Could you check a few things on this model? Use its own coordinates, in mm. Face numbers are marked on the shaded views. A direction names the side the tool comes from. Coordinates: 2 decimals unless noted, no trailing zeros. Loops run counter-clockwise (first coordinate to the right, second up) from the corner with the lowest first, then second, coordinate; pieces in that order, holes last. Notation, with made-up numbers: (-8, 87.5) - (36, 87.5) arc R9 ccw to (36, 95.5) - close; hole circle Ø9 at (29, -38.75). An arc over 180 degrees is marked (long way). Put each result on its own line as item: value. Start each with the question number.
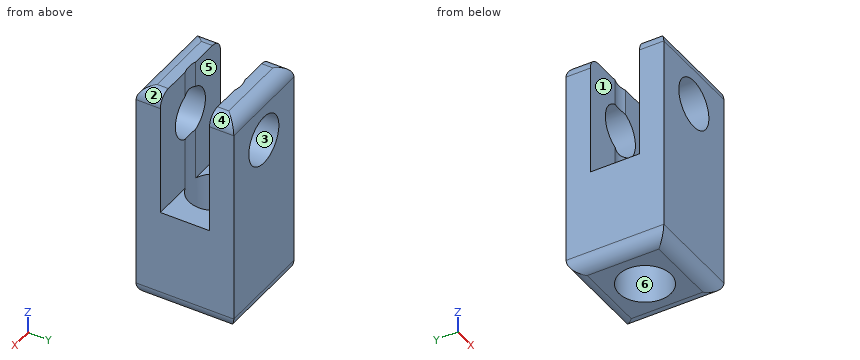
```python
from build123d import *

# Parameters (mm, degrees)
SKETCH1_W           = 19.05
SKETCH1_H           = 19.05
BOSS_EXTRUDE1_DEPTH = 43.18
FILLET1_R           = 2.54
CUT_EXTRUDE1_REACH  = 45.18
SKETCH2_R           = 5.08
SKETCH3_W           = 43.18
SKETCH3_H           = 9.6012
CUT_EXTRUDE2_DEPTH  = 20.05
SKETCH4_R           = 4.7625
CUT_EXTRUDE3_DEPTH  = 20.05


with BuildPart() as part:
    # Sketch1 → Boss-Extrude1 (new body)
    with BuildSketch(Plane.XY):
        with Locations((9.525, 9.525)):
            Rectangle(SKETCH1_W, SKETCH1_H)
    extrude(amount=BOSS_EXTRUDE1_DEPTH)

    # Fillet1
    fillet1_edges = [part.edges().sort_by_distance(p)[0] for p in [
        (19.05, 9.525, 43.18),
        (9.525, 19.05, 43.18),
        (0, 9.525, 43.18),
        (9.525, 19.05, 0),
        (19.05, 9.525, 0),
        (9.525, 0, 0),
        (0, 9.525, 0),
        (9.525, 0, 43.18),
    ]]
    fillet(fillet1_edges, radius=FILLET1_R)

    # Sketch2 → Cut-Extrude1 (cut, up to next)
    with BuildSketch(Plane(origin=(0, 0, 0), x_dir=(-1, 0, 0), z_dir=(0, 0, -1)), mode=Mode.PRIVATE) as cut_extrude1_sk1:
        with Locations((-9.525, 9.525)):
            Circle(SKETCH2_R)
    cut_extrude1_tool1 = extrude(cut_extrude1_sk1.sketch, amount=-CUT_EXTRUDE1_REACH, mode=Mode.PRIVATE) & part.part
    add(cut_extrude1_tool1.solids().sort_by_distance((9.525, 9.525, 0))[0], mode=Mode.SUBTRACT)

    # Sketch3 → Cut-Extrude2 (cut, through all)
    with BuildSketch(Plane(origin=(19.05, 0, 0), x_dir=(0, 0, -1), z_dir=(1, 0, 0))):
        with Locations((-40.64, 9.525)):
            Rectangle(SKETCH3_W, SKETCH3_H)
    extrude(amount=-CUT_EXTRUDE2_DEPTH, mode=Mode.SUBTRACT)

    # Sketch4 → Cut-Extrude3 (cut, through all)
    with BuildSketch(Plane.XZ):
        with Locations((9.525, 33.655)):
            Circle(SKETCH4_R)
    extrude(amount=-CUT_EXTRUDE3_DEPTH, mode=Mode.SUBTRACT)


solid = part.part
```
(1) I want a section at D-D on x = 3.25. List the corners of the cut face in (y, z) for me.
(2) Which directions (+Z, -Z, +X, -X, +Y, -Y) give clear straight access to the entire face, cutting with the end or side of a thin tool? Please do the marked faces 1 and 2.
(3) If we mould it in two halves opening along X, with no side actions, what happens to the marked faces 3, 4, 5 and 6? For each: pulls with the +X half, pulls with the -X half, needs draft (parallel to the pull), parting line crosses it, or undercut.
(4) I want a section at B-B on x = 7.25. List the corners of the cut face in (y, z) for me, and give its area (3 significant figures).
(5) I want a section at A-A on z = 22. List the corners of the cut face in (x, y) for me (3 decimals), and give its area (3 significant figures).
(6) I want a section at C-C on y = 5.75. List the corners of the cut face in (x, z) for me.
(7) I need wall thicknesses on L1, parallel to Y at x = 3.5, z = 32; L2, parallel to Y at x = 5.75, z = 2.5; L3, parallel to X at y = 16.5, z = 32.5. Which ranges of each line are inside material? Lowest first, please. Write a range as [from, to].
Answer sheet:
1. outline: (0, 2.54) arc R2.54 ccw to (2.54, 0) - (16.51, 0) arc R2.54 ccw to (19.05, 2.54) - (19.05, 40.64) arc R2.54 ccw to (16.51, 43.18) - (14.33, 43.18) - (14.33, 19.05) - (4.72, 19.05) - (4.72, 43.18) - (2.54, 43.18) arc R2.54 ccw to (0, 40.64) - close
2. face 1: +Z, +X, -X
2. face 2: +Z, +X, +Y, -Y
3. face 3: undercut
3. face 4: pulls with the +X half
3. face 5: needs draft
3. face 6: undercut
4. outline: (0, 2.54) arc R2.54 ccw to (2.54, 0) - (4.98, 0) - (4.98, 19.05) - (4.72, 19.05) - (4.72, 29.47) - (0, 29.47) - close; (0, 37.84) - (4.72, 37.84) - (4.72, 43.18) - (2.54, 43.18) arc R2.54 ccw to (0, 40.64) - close; (14.07, 0) - (16.51, 0) arc R2.54 ccw to (19.05, 2.54) - (19.05, 29.47) - (14.33, 29.47) - (14.33, 19.05) - (14.07, 19.05) - close; (14.33, 37.84) - (19.05, 37.84) - (19.05, 40.64) arc R2.54 ccw to (16.51, 43.18) - (14.33, 43.18) - close
4. area: 333 mm^2
5. outline: (0, 0) - (19.05, 0) - (19.05, 4.724) - (11.187, 4.724) arc R5.08 cw to (7.863, 4.724) - (0, 4.724) - close; (0, 14.326) - (7.863, 14.326) arc R5.08 cw to (11.187, 14.326) - (19.05, 14.326) - (19.05, 19.05) - (0, 19.05) - close
5. area: 179 mm^2
6. outline: (0, 2.54) arc R2.54 ccw to (2.54, 0) - (6.13, 0) - (6.13, 19.05) - (0, 19.05) - close; (12.92, 0) - (16.51, 0) arc R2.54 ccw to (19.05, 2.54) - (19.05, 19.05) - (12.92, 19.05) - close
7. L1: y = [0, 4.72], [14.33, 19.05]
7. L2: y = [0, 6.13], [12.92, 19.05]
7. L3: x = [0, 4.9], [14.15, 19.05]
